The model under review builds one solid part; all positions refer to its coordinate system, in mm. A direction names the side the tool comes from. Give positions to 0.01 mm unless a question says otherwise; leave off trailing zeros. Write each loop counter-clockwise with the first axis right and the second up, starting at its lowest first coordinate (ties: lowest second). Pieces come first, ordered by that corner, then holes. Notation, with made-up numbers: (-39, 0.25) -> (6, 0.25) arc R23 cw to (6, 27.25) -> close; hole circle Ø2 at (13.25, 78.25). An arc over 180 degrees is marked (long way). Use CSV: the item, a comma, the result in double quotes.
```python
from build123d import *

# Parameters (mm, degrees)
BOSS_EXTRUDE1_DEPTH                             = 7.366
BOSS_EXTRUDE1_DEPTH_BACK                        = 19.431
SKETCH1_R                                       = 11.9888
SKETCH3_W                                       = 26.0096
SKETCH3_H                                       = 31.0388
BOSS_EXTRUDE3_DEPTH                             = 4.699
CSK_FOR_M3_FLAT_HEAD_MACHINE_SCREW2_D           = 3.4
CSK_FOR_M3_FLAT_HEAD_MACHINE_SCREW2_CSINK_D     = 6.3
CSK_FOR_M3_FLAT_HEAD_MACHINE_SCREW2_CSINK_ANGLE = 90
SKETCH11_R                                      = 9.1186
SKETCH11_R_2                                    = 6.5786
CUT_EXTRUDE1_DEPTH                              = 21.717
FILLET1_R                                       = 2.54
SKETCH12_R                                      = 2.921
CUT_EXTRUDE3_DEPTH                              = 21.717
BOSS_EXTRUDE4_DEPTH                             = 9.525
SKETCH14_W                                      = 4.7625
SKETCH14_H                                      = 0.508
SKETCH14_W_2                                    = 0.508
SKETCH14_H_2                                    = 4.7625
BOSS_EXTRUDE5_DEPTH                             = 7.62
FILLET2_R                                       = 1.27


with BuildPart() as part:
    # Sketch1 → Boss-Extrude1 (new, two sides: drawn at the far end of the back side and taken through both)
    with BuildSketch(Plane(origin=(0, 0, 0), x_dir=(1, 0, 0), z_dir=(0, 1, 0)).offset(-BOSS_EXTRUDE1_DEPTH_BACK)):
        with Locations(Location((0, 0, 0), (0, 0, 270))):
            Circle(SKETCH1_R)
    extrude(amount=BOSS_EXTRUDE1_DEPTH + BOSS_EXTRUDE1_DEPTH_BACK)

    # Sketch3 → Boss-Extrude3 (add)
    with BuildSketch(Plane(origin=(0, 0, 0), x_dir=(1, 0, 0), z_dir=(0, 1, 0))):
        Rectangle(SKETCH3_W, SKETCH3_H)
    extrude(amount=BOSS_EXTRUDE3_DEPTH)

    # CSK for M3 Flat Head Machine Screw2 (through all)
    with Locations(Plane(origin=(0, 4.699, 0), x_dir=(1, 0, 0), z_dir=(0, 1, 0))):
        with Locations((-9.5758, 12.0904), (9.5758, -12.0904)):
            CounterSinkHole(CSK_FOR_M3_FLAT_HEAD_MACHINE_SCREW2_D / 2, CSK_FOR_M3_FLAT_HEAD_MACHINE_SCREW2_CSINK_D / 2, counter_sink_angle=CSK_FOR_M3_FLAT_HEAD_MACHINE_SCREW2_CSINK_ANGLE)

    # Sketch11 → Cut-Extrude1 (cut)
    with BuildSketch(Plane(origin=(0, 7.366, 0), x_dir=(1, 0, 0), z_dir=(0, 1, 0))):
        with Locations(Location((0, 0, 0), (0, 0, 270))):
            Circle(SKETCH11_R)
        with Locations(Location((0, 0, 0), (0, 0, 270))):
            Circle(SKETCH11_R_2, mode=Mode.SUBTRACT)
    extrude(amount=-CUT_EXTRUDE1_DEPTH, mode=Mode.SUBTRACT)

    # Fillet1
    fillet1_edges = [part.edges().sort_by_distance(p)[0] for p in [
        (13.0048, 2.3495, -15.5194),
        (-13.0048, 2.3495, -15.5194),
        (-13.0048, 2.3495, 15.5194),
        (13.0048, 2.3495, 15.5194),
    ]]
    fillet(fillet1_edges, radius=FILLET1_R)

    # Sketch12 → Cut-Extrude3 (cut)
    with BuildSketch(Plane(origin=(0, 7.366, 0), x_dir=(1, 0, 0), z_dir=(0, 1, 0))):
        with Locations(Location((0, 0, 0), (0, 0, 270))):
            Circle(SKETCH12_R)
    extrude(amount=-CUT_EXTRUDE3_DEPTH, mode=Mode.SUBTRACT)

    # Sketch13 → Boss-Extrude4 (add)
    with BuildSketch(Plane.XZ.offset(19.431)):
        Polygon((3.175, 0.36195), (-3.175, 0.36195), (-3.175, 8.61695), (-3.8989, 8.61695), (-3.8989, 4.4069), (-8.9789, 4.4069), (-8.9789, 3.683), (-3.8989, 3.683), (-3.8989, -3.683), (-8.9789, -3.683), (-8.9789, -4.4069), (-3.8989, -4.4069), (-3.8989, -8.61695), (-3.175, -8.61695), (-3.175, -0.36195), (3.175, -0.36195), (3.175, -8.61695), (3.8989, -8.61695), (3.8989, -4.4069), (8.9789, -4.4069), (8.9789, -3.683), (3.8989, -3.683), (3.8989, 3.683), (8.9789, 3.683), (8.9789, 4.4069), (3.8989, 4.4069), (3.8989, 8.61695), (3.175, 8.61695), align=None)
    extrude(amount=BOSS_EXTRUDE4_DEPTH)

    # Sketch14 → Boss-Extrude5 (add)
    with BuildSketch(Plane.XZ.offset(19.431)):
        with Locations((0, 3.79095)):
            Rectangle(SKETCH14_W, SKETCH14_H)
        with Locations((-6.0579, 0)):
            Rectangle(SKETCH14_W_2, SKETCH14_H_2)
        with Locations((6.0579, 0)):
            Rectangle(SKETCH14_W_2, SKETCH14_H_2)
    extrude(amount=BOSS_EXTRUDE5_DEPTH)

    # Fillet2
    fillet2_edges = [part.edges().sort_by_distance(p)[0] for p in [
        (0, -19.431, -11.9888),
    ]]
    fillet(fillet2_edges, radius=FILLET2_R)


solid = part.part
```
Q1. Consider section C-C (y = -23). State how many separate pieces and enclosed holes the cut face has, then the cut area to 3 significant figures.
Derived:
separate pieces,"4"
enclosed holes,"0"
area,"51.5 mm2"
Q2. Insertion check: pin 1 (5 mm diameter, centred on x = 0.5, y = -24, fed in from -Z); pin 2 (0.6 mm diameter, centred on x = 6, z = -0.5, fed in from -Y); pin 3 (1.5 mm diameter, centred on x = -6, y = -22.5, fed in from -Z). Each pin has a flat end and moves straight along its axis. Give the tip position at first contact, or say it passes through.
Derived:
pin 1,"stops at z = -0.36"
pin 2,"stops at y = -27.05"
pin 3,"stops at z = -4.41"
Q3. Consider section B-B (y = 0.5). Write out the cut boundary in (x, z).
Derived:
outline,"(-13, -12.98) arc R2.54 ccw to (-10.46, -15.52) -> (10.46, -15.52) arc R2.54 ccw to (13, -12.98) -> (13, 12.98) arc R2.54 ccw to (10.46, 15.52) -> (-10.46, 15.52) arc R2.54 ccw to (-13, 12.98) -> close; circle Ø13.16 at (0, 0); hole circle Ø3.4 at (-9.58, -12.09); hole circle Ø18.24 at (0, 0); hole circle Ø5.84 at (0, 0); hole circle Ø3.4 at (9.58, 12.09)"
Q4. The part is to be moulded in two halves that separate along X. For faces 1 (the flat face through (0, -28.956, 0)), 2 (the flat face through (-6.312, -23, 0)), 3 (the flat face through (0, -24, -0.362)), say which applies: pulls with the +X half, pulls with the -X half, needs draft (parallel to the pull), parting line crosses it, or undercut.
Derived:
face 1,"needs draft"
face 2,"pulls with the -X half"
face 3,"undercut"
Q5. To check wall thickness, follow probe 1 along X at (y, z) = (2.5, 0); probe 2 along X at (y, z) = (-6, 0); probe 3 along X at (y, z) = (-23.5, 3.5) (3 decimals). State the ranges of each line that lie inside material, in increasing order.
Derived:
probe 1,"x = -13 to -9.12, -6.58 to -2.92, 2.92 to 6.58, 9.12 to 13"
probe 2,"x = -11.99 to -9.12, -6.58 to -2.92, 2.92 to 6.58, 9.12 to 11.99"
probe 3,"x = -3.899 to -3.175, 3.175 to 3.899"
Q6. Machinability: for faces 4 (the flat face through (6, -24, -3.683)), 5 (the flat face through (5.804, -23, 0)), 6 (the flat face through (-3.899, -24, -6)), which of the approach directions +Z, -Z, +X, -X, +Y, -Y give a long, thin tool a straight path to every point of the face, cutting with its end or side? Answer none if there is none.
Derived:
face 4,"+X, -Y"
face 5,"-Y"
face 6,"-Z, -X, -Y"
